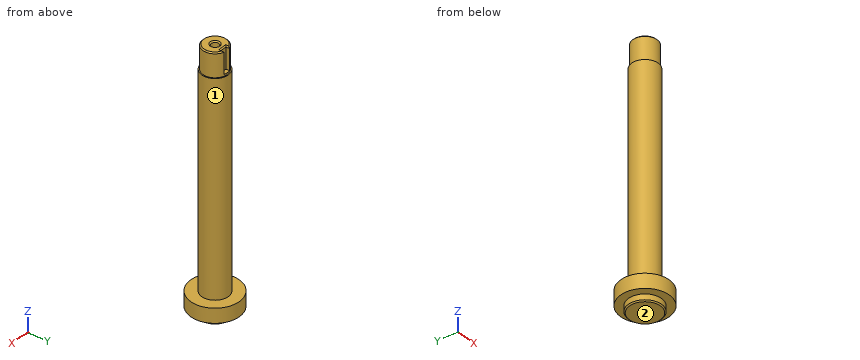
```python
from build123d import *

# Parameters (mm, degrees)
SKETCH1_W                      = 22
SKETCH1_H                      = 13
SKETCH2_R                      = 12
BOSS_EXTRUDE1_DEPTH            = 190
SKETCH3_R                      = 11
BOSS_EXTRUDE2_DEPTH            = 21.5
CUT_EXTRUDE1_START             = -20
CUT_EXTRUDE1_DEPTH             = 20
SKETCH5_R                      = 15
BOSS_EXTRUDE3_DEPTH            = 6
F_6_8_6_8_DIAMETER_HOLE1_D     = 6.8
F_6_8_6_8_DIAMETER_HOLE1_DEPTH = 16
CHAMFER1_SIZE                  = 1


with BuildPart() as part:
    # Sketch1 → Revolve1 (revolve)
    with BuildSketch(Plane.XZ, mode=Mode.PRIVATE) as revolve1_sk:
        with Locations((11, 12.5)):
            Rectangle(SKETCH1_W, SKETCH1_H)
    revolve(revolve1_sk.sketch.rotate(Axis((0, 0, 19), (0, 0, -1)), 180), axis=Axis((0, 0, 19), (0, 0, -1)))

    # Sketch2 → Boss-Extrude1 (add)
    with BuildSketch(Plane.XY.offset(19)):
        Circle(SKETCH2_R)
    extrude(amount=BOSS_EXTRUDE1_DEPTH)

    # Sketch3 → Boss-Extrude2 (add)
    with BuildSketch(Plane.XY.offset(209)):
        Circle(SKETCH3_R)
    extrude(amount=BOSS_EXTRUDE2_DEPTH)

    # Sketch4 → Cut-Extrude1 (cut)
    with BuildSketch(Plane.XY.offset(230.5).offset(CUT_EXTRUDE1_START)):
        with BuildLine():
            Line((3, 7.5), (3, 10.583005244))
            ThreePointArc((3, 10.583005244), (0, 11), (-3, 10.583005244))
            Line((-3, 10.583005244), (-3, 7.5))
            Line((-3, 7.5), (3, 7.5))
        make_face()
    extrude(amount=CUT_EXTRUDE1_DEPTH, mode=Mode.SUBTRACT)

    # Sketch5 → Boss-Extrude3 (add)
    with BuildSketch(Plane(origin=(0, 0, 6), x_dir=(-1, 0, 0), z_dir=(0, 0, -1))):
        with Locations(Location((0, 0, 0), (0, 0, 90))):
            Circle(SKETCH5_R)
    extrude(amount=BOSS_EXTRUDE3_DEPTH)

    # Ø6.8 (6.8) Diameter Hole1
    with Locations(Plane.XY.offset(230.5)):
        with Locations((0, 0)):
            Hole(F_6_8_6_8_DIAMETER_HOLE1_D / 2, depth=F_6_8_6_8_DIAMETER_HOLE1_DEPTH)

    # Chamfer1
    chamfer1_edges = [part.edges().sort_by_distance(p)[0] for p in [
        (-6.633249581, -8.774964387, 230.5),
        (0, 7.5, 230.5),
        (3, 9.041502622, 230.5),
        (-3, 9.041502622, 230.5),
        (0, -15, 0),
        (3.4, 0, 230.5),
    ]]
    chamfer(chamfer1_edges, length=CHAMFER1_SIZE)


solid = part.part
```
Build history of the part. All positions in model axes, mm. Face numbers are marked on the shaded views. A direction names the side the tool comes from. Round coordinates to 2 decimals unless told otherwise and drop trailing zeros. Write each loop counter-clockwise with the first axis right and the second up, starting at its lowest first coordinate (ties: lowest second). Pieces come first, ordered by that corner, then holes.
1) Band-saw the part on C-C, the plane y = -18.5. List the corners of the cut face in (x, z), and give its area (3 significant figures).
2) Band-saw the part on A-A, the plane x = 0. List the corners of the cut face in (y, z), and give its area (3 significant figures).
3) Drill centre lines: probe 1 along Y at (x, z) = (0, 220.25); probe 2 along Z at (x, y) = (13, 16.5); probe 3 along Z at (x, y) = (-6.5, 12). Where is each one in solid material? Low to high.
4) 3-axis set-ups, long thin cutter, end or side, ignore diameter. For the marked faces 1 and 2: which of +Z, -Z, +X, -X, +Y, -Y reach the whole face in a straight line?
5) Band-saw the part on B-B, the plane z = 143. List the corners of the cut face in (x, y).
6) Pin check, flat tips, straight feed: pin 1 (1.7 mm diameter, centred on x = 1.5, y = 10, fed in from +Z); pin 2 (8 mm diameter, centred on y = -0.5, z = 153, fed in from -X); pin 3 (8 mm diameter, centred on x = 3, z = 158, fed in from +Y). Stop position of each tip, or through.
Ans:
1. outline: (-11.91, 6) - (11.91, 6) - (11.91, 19) - (-11.91, 19) - close
1. area: 310 mm2
2. outline: (-22, 6) - (-15, 6) - (-15, 1) - (-14, 0) - (14, 0) - (15, 1) - (15, 6) - (22, 6) - (22, 19) - (12, 19) - (12, 209) - (11, 209) - (11, 210.5) - (7.5, 210.5) - (7.5, 229.5) - (6.5, 230.5) - (4.4, 230.5) - (3.4, 229.5) - (3.4, 214.5) - (-3.4, 214.5) - (-3.4, 229.5) - (-4.4, 230.5) - (-10, 230.5) - (-11, 229.5) - (-11, 209) - (-12, 209) - (-12, 19) - (-22, 19) - close
2. area: 5,600 mm2
3. probe 1: y = -11 to -3.4, 3.4 to 7.5
3. probe 2: z = 6 to 19
3. probe 3: z = 0 to 19
4. face 1: +Z
4. face 2: -Z, +X, -X, +Y, -Y
5. outline: circle Ø24 at (0, 0)
6. pin 1: stops at z = 210.5
6. pin 2: stops at x = -12
6. pin 3: stops at y = 12
